Geometry: final body of the model. Coordinates: model frame, mm. Face numbers are marked on the shaded views. A direction names the side the tool comes from. Give positions to 0.01 mm unless a question says otherwise; leave off trailing zeros. Order: outer loops, then holes, each group sorted by start corner. A loop starts at its lowest first (then second) coordinate and runs counter-clockwise, first axis right, second up. Notation, with made-up numbers: (-34, 29.5) - (19, 29.5) arc R24 ccw to (19, 42.5) - close; hole circle Ø2 at (-29, 18.25). An arc over 180 degrees is marked (long way). Put each result on its own line as item: value. Start each with the question number.
1. First-contact query: P1, Ø2.5, axis at x = 0, z = 6, coming from the -Y side; P2, Ø4.5, axis at x = 0.5, z = 6, coming from the +Y side; P3, Ø2, axis at y = 1.5, z = -3, coming from the +X side; P4, Ø1, axis at x = -8.5, y = 5.5, coming from the +Z side. Flat tips, straight axial feed; report the tip coordinate or a pass-through.
2. Ray query, line 1 along Z through (x, y) = (1.25, 1.25); line 2 along Z through (x, y) = (2, 5); line 3 along X through (y, z) = (3.75, -5). Return the intervals inside material, ascending. Write a range as from..to.
3. Section C-C on y = 1. Return the cut outline in (x, z), plus the area to 3 significant figures.
4. Section A-A on x = 0. Return the cut outline in (y, z).
5. Set-up query: the marked faces 1 and 2. Return all of +Z, -Z, +X, -X, +Y, -Y with unobstructed straight access to the full face (end or side cutting, diameter ignored); none if empty.
6. Section B-B on y = 4.5. Return the cut outline in (x, z).
7. Mould query, pull axis X, two halves, no side actions, for the marked faces 3, 4 and 5. Classes: pulls with the +X half, pulls with the -X half, needs draft (parallel to the pull), parting line crosses it, or undercut.
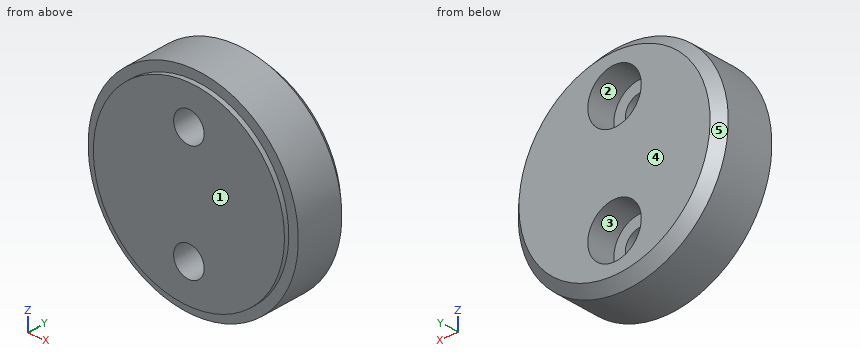
from build123d import *

# Parameters (mm, degrees)
ESQUISSE1_R             = 10
BOSS_EXTRU_1_DEPTH      = 0.5
ESQUISSE2_R             = 11
BOSS_EXTRU_2_DEPTH      = 6
CHANFREIN1_SIZE         = 1
ESQUISSE3_R             = 1.6
ENL_V_MAT_EXTRU_1_DEPTH = 17.8597153
ESQUISSE4_R             = 2.8
ENL_V_MAT_EXTRU_2_DEPTH = 3


with BuildPart() as part:
    # Esquisse1 → Boss.-Extru.1 (new body)
    with BuildSketch(Plane(origin=(0, 0, 0), x_dir=(1, 0, 0), z_dir=(0, 1, 0))):
        with Locations(Location((0, 0, 0), (0, 0, 270))):
            Circle(ESQUISSE1_R)
    extrude(amount=BOSS_EXTRU_1_DEPTH)

    # Esquisse2 → Boss.-Extru.2 (add)
    with BuildSketch(Plane(origin=(0, 0.5, 0), x_dir=(1, 0, 0), z_dir=(0, 1, 0))):
        with Locations(Location((0, 0, 0), (0, 0, 270))):
            Circle(ESQUISSE2_R)
    extrude(amount=BOSS_EXTRU_2_DEPTH)

    # Chanfrein1
    chanfrein1_edges = [part.edges().sort_by_distance(p)[0] for p in [
        (0, 6.5, -11),
    ]]
    chamfer(chanfrein1_edges, length=CHANFREIN1_SIZE)

    # Esquisse3 → Enlèv. mat.-Extru.1 (cut, through all)
    with BuildSketch(Plane(origin=(0, 6.5, 0), x_dir=(1, 0, 0), z_dir=(0, 1, 0))):
        with Locations(Location((0, 6, 0), (0, 0, 270))):
            Circle(ESQUISSE3_R)
        with Locations(Location((0, -6, 0), (0, 0, 270))):
            Circle(ESQUISSE3_R)
    extrude(amount=-ENL_V_MAT_EXTRU_1_DEPTH, mode=Mode.SUBTRACT)

    # Esquisse4 → Enlèv. mat.-Extru.2 (cut)
    with BuildSketch(Plane(origin=(0, 6.5, 0), x_dir=(1, 0, 0), z_dir=(0, 1, 0))):
        with Locations(Location((0, 6, 0), (0, 0, 270))):
            Circle(ESQUISSE4_R)
        with Locations(Location((0, -6, 0), (0, 0, 270))):
            Circle(ESQUISSE4_R)
    extrude(amount=-ENL_V_MAT_EXTRU_2_DEPTH, mode=Mode.SUBTRACT)


solid = part.part
Resolved:
1. P1: through
1. P2: y = 3.5
1. P3: x = 10.82
1. P4: z = 7.55
2. line 1: -10.93..-7, -5..5, 7..10.93
2. line 2: -10.82..-7.96, -4.04..4.04, 7.96..10.82
2. line 3: -9.8..-2.62, 2.62..9.8
3. outline: circle Ø22 at (0, 0); hole circle Ø3.2 at (0, -6); hole circle Ø3.2 at (0, 6)
3. area: 364 mm^2
4. outline: (0, -10) - (0.5, -10) - (0.5, -11) - (5.5, -11) - (6.5, -10) - (6.5, -8.8) - (3.5, -8.8) - (3.5, -7.6) - (0, -7.6) - close; (0, -4.4) - (3.5, -4.4) - (3.5, -3.2) - (6.5, -3.2) - (6.5, 3.2) - (3.5, 3.2) - (3.5, 4.4) - (0, 4.4) - close; (0, 7.6) - (3.5, 7.6) - (3.5, 8.8) - (6.5, 8.8) - (6.5, 10) - (5.5, 11) - (0.5, 11) - (0.5, 10) - (0, 10) - close
5. face 1: +Z, -Z, +X, -X, -Y
5. face 2: +Y
6. outline: circle Ø22 at (0, 0); hole circle Ø5.6 at (0, -6); hole circle Ø5.6 at (0, 6)
7. face 3: undercut
7. face 4: needs draft
7. face 5: parting line crosses it
